```python
from build123d import *

# Parameters (mm, degrees)
F0_W     = 155
F0_H     = 12.5
F0_W_2   = 8
F0_H_2   = 15
F0_W_3   = 10
F0_H_3   = 30
F1_DEPTH = 15
F2_R     = 2


with BuildPart() as f1:
    # F0 (on Top) → F1 (new body)
    with BuildSketch(Plane.XY):
        with Locations((-59.8887689211, 33.75)):
            Rectangle(F0_W, F0_H)
        Polygon((17.6112310789, 27.5), (-137.3887689211, 27.5), (-137.3887689211, 15), (-127.3887689211, 15), (-117.3887689211, 15), (-109.3887689211, 15), (-99.3887689211, 15), (-85.3887689211, 15), (17.6112310789, 15), align=None)
        with BuildLine():
            ThreePointArc((17.6112310789, 15), (85.3029731554, 27.5), (17.6112310789, 40))
            Line((17.6112310789, 40), (17.6112310789, 27.5))
            Line((17.6112310789, 27.5), (17.6112310789, 15))
        make_face()
        with BuildLine():
            ThreePointArc((67.8029731554, 27.5), (50.3029731554, 10), (32.8029731554, 27.5))
            ThreePointArc((32.8029731554, 27.5), (50.3029731554, 45), (67.8029731554, 27.5))
        make_face(mode=Mode.SUBTRACT)
        Polygon((-92.3888981342, 0), (-85.3887689211, 15), (-99.3887689211, 15), align=None)
        with Locations((-113.3887689211, 7.5)):
            Rectangle(F0_W_2, F0_H_2)
        with Locations((-132.3887689211, 0)):
            Rectangle(F0_W_3, F0_H_3)
    extrude(amount=F1_DEPTH)

    # F2
    f2_edges = [f1.edges().sort_by_distance(p)[0] for p in [
        (-59.888769, 40, 15),
        (85.302973, 27.5, 15),
        (-33.888769, 15, 15),
        (-88.888834, 7.5, 15),
        (-122.388769, 15, 15),
        (-109.388769, 7.5, 15),
        (-132.388769, -15, 15),
        (-127.388769, 0, 15),
        (-137.388769, 12.5, 15),
        (-113.388769, 0, 15),
        (-117.388769, 7.5, 15),
        (-95.888834, 7.5, 15),
        (67.802973, 27.5, 15),
        (-104.388769, 15, 15),
    ]]
    fillet(f2_edges, radius=F2_R)


solid = f1.part
```
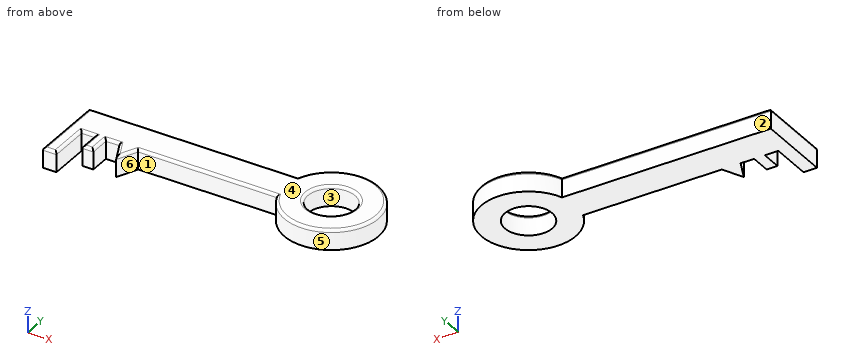
Source: CAD feature listing. Evaluate the final solid. Frame: model axes, mm. Face numbers are marked on the shaded views. A direction names the side the tool comes from. Coordinates: 2 decimals unless noted, no trailing zeros. Order: outer loops, then holes, each group sorted by start corner. A loop starts at its lowest first (then second) coordinate and runs counter-clockwise, first axis right, second up. Notation, with made-up numbers: (87.5, 41.5) - (132.5, 41.5) arc R31 ccw to (132.5, 76.5) - close; hole circle Ø6 at (37, -24). An arc over 180 degrees is marked (long way). One line per item, written item: value.
1) Contact query for flat-ended pins moving along their axis: pin 1 (4 mm diameter, centred on y = 2.5, z = 4.5, fed in from +X); pin 2 (4 mm diameter, centred on x = -63.5, z = 9.5, fed in from +Y); pin 3 (9 mm diameter, centred on x = -113.5, z = 5, fed in from -Y). Output: stop coordinate, or through.
Computed values:
pin 1: stops at x = 76.68
pin 2: stops at y = 40
pin 3: stops at y = 0
2) Reachability of the marked faces 1, 2 and 3 from +Z, -Z, +X, -X, +Y, -Y: full face, straight path, thin tool, end or side. Return the list, or none.
Computed values:
face 1: +Z, -Z, -Y
face 2: +Z, -Z, -X, +Y
face 3: +Z, -Z
3) Ray query, line 1 (X direction, y = 2, z = 6); line 2 (X direction, y = 37, z = 9.5); line 3 (X direction, y = 39.5, z = 4). Return the intervals inside material, ascending. Write a range as [from, to].
Computed values:
line 1: x = [-137.39, -127.39], [-117.39, -109.39], [-93.32, -91.46], [26.33, 74.28]
line 2: x = [-137.39, 35.61], [65, 83.99]
line 3: x = [-137.39, 37.57], [63.04, 83.18]
4) Cut plane B-B on x = -63. Output: boundary loops of the cut face in (y, z), plus the area to 3 significant figures.
Computed values:
outline: (15, 0) - (40, 0) - (40, 13) arc R2 ccw to (38, 15) - (17, 15) arc R2 ccw to (15, 13) - close
area: 373 mm^2
5) Cut plane A-A on z = 11. Output: boundary loops of the cut face in (x, y).
Computed values:
outline: (-137.39, -15) - (-127.39, -15) - (-127.39, 15) - (-117.39, 15) - (-117.39, 0) - (-109.39, 0) - (-109.39, 15) - (-99.39, 15) - (-92.39, 0) - (-85.39, 15) - (17.61, 15) arc R35 ccw (long way) to (17.61, 40) - (-137.39, 40) - close; hole circle Ø35 at (50.3, 27.5)
6) Mould query, pull axis X, two halves, no side actions, for the marked faces 4, 5 and 6. Classes: released by +X, released by -X, zero draft, split by the parting line, or undercut.
Computed values:
face 4: zero draft
face 5: undercut
face 6: undercut
